Here's how the part is built. I have some questions about the finished solid (model axes, mm). A direction names the side the tool comes from. Coordinates: 2 decimals unless noted, no trailing zeros. Write each loop counter-clockwise with the first axis right and the second up, starting at its lowest first coordinate (ties: lowest second). Pieces come first, ordered by that corner, then holes. Notation, with made-up numbers: (-23, 41.5) -> (17, 41.5) arc R25 ccw to (17, 72.5) -> close; hole circle Ø2 at (6, 72). An arc over 180 degrees is marked (long way). Use a Markdown table: item, result. Add a question column.
Item 1: Imagine slicing it at C-C, the plane z = 16. Write out the boundary of the cut face in (x, y).
Item 2: Imagine slicing it at D-D, the plane z = 33.5. Write out the boundary of the cut face in (x, y), and give its area (3 significant figures).
Item 3: On a 3-axis mill with a long thin cutter (end or side, diameter ignored), from which of +Z, -Z, +X, -X, +Y, -Y can I reach the whole of each face in a straight line? I mean faces 1 (the flat face through (-45, 60, -15)), 2 (the flat face through (-6.604, 44.79, 42.767)). Say none if no direction works.
Item 4: If I drill on line 1 along Z through (x, y) = (22.5, 42.5); line 2 along X through (y, z) = (48, 29.5); line 3 along Z through (x, y) = (22, 42), over which ranges is the centre line in solid material (lowest first)? Write a range as from..to.
Item 5: Will these pins go through, and if not, where does the flat tip stop? pin 1 Ø21 at (x, z) = (-36, 9.5) entering from +Y; pin 2 Ø2 at (x, y) = (-26, 18) entering from +Z; pin 3 Ø1 at (x, y) = (1, 31.5) entering from -Z; pin 4 Ø5 at (x, y) = (-27, 41.5) entering from +Z.
Item 6: Imagine slicing it at A-A, the plane y = 54. Count the separate pieces of the cut face and the enclosed holes in it, and give its area (3 significant figures).
Item 7: Imagine slicing it at B-B, the plane y = 17.5. Write out the boundary of the cut face in (x, z), and give its area (3 significant figures).
Item 8: If we mould it in two halves opening along X, with no side actions, what happens to faces 3 (the flat face through (-33.736, 44.79, -27.102)), 4 (the flat face through (35, 60, -35)), 5 (the flat face through (-40.339, 44.79, 15.665))? For each: pulls with the +X half, pulls with the -X half, needs draft (parallel to the pull), parting line crosses it, or undercut.
```python
from build123d import *

# Parameters (mm, degrees)
BOSS_EXTRUDE1_DEPTH   = 60
BOSS_EXTRUDE1_2_DEPTH = 60
BOSS_EXTRUDE1_3_DEPTH = 60
BOSS_EXTRUDE1_4_DEPTH = 60
BOSS_EXTRUDE1_5_DEPTH = 60
BOSS_EXTRUDE1_6_DEPTH = 60
BOSS_EXTRUDE2_DEPTH   = 30


with BuildPart() as part:
    # Sketch2 → Boss-Extrude1 (new body)
    with BuildSketch(Plane(origin=(0, 0, 0), x_dir=(1, 0, 0), z_dir=(0, 1, 0))):
        with BuildLine():
            Line((18.030501156, -69.282032303), (39.961980888, -47.664077799))
            Line((39.961980888, -47.664077799), (13.634472037, -20.954741045))
            ThreePointArc((13.634472037, -20.954741045), (6.29646333, -24.194101544), (-1.689726767, -24.942831103))
            Line((-1.689726767, -24.942831103), (-11.656936488, -61.097790964))
            Line((-11.656936488, -61.097790964), (18.030501156, -69.282032303))
        make_face()
    extrude(amount=BOSS_EXTRUDE1_DEPTH)



with BuildPart() as body_2:
    # Sketch2 → Boss-Extrude1 2 (new body)
    with BuildSketch(Plane(origin=(0, 0, 0), x_dir=(1, 0, 0), z_dir=(0, 1, 0))):
        with BuildLine():
            Line((-21.297311778, -58.440129534), (-11.330102056, -22.285169674))
            ThreePointArc((-11.330102056, -22.285169674), (-17.804474894, -17.54994797), (-22.445988761, -11.008069246))
            Line((-22.445988761, -11.008069246), (-58.740707334, -20.453692353))
            Line((-58.740707334, -20.453692353), (-50.984749422, -50.255888195))
            Line((-50.984749422, -50.255888195), (-21.297311778, -58.440129534))
        make_face()
    extrude(amount=BOSS_EXTRUDE1_2_DEPTH)


with BuildPart() as body_3:
    # Sketch2 → Boss-Extrude1 3 (new body)
    with BuildSketch(Plane(origin=(0, 0, 0), x_dir=(1, 0, 0), z_dir=(0, 1, 0))):
        with BuildLine():
            ThreePointArc((-24.964574093, -1.330428629), (-24.100938224, 6.644153574), (-20.756261995, 13.934761857))
            Line((-20.756261995, 13.934761857), (-47.083770846, 40.644098611))
            Line((-47.083770846, 40.644098611), (-69.015250578, 19.026144108))
            Line((-69.015250578, 19.026144108), (-61.259292666, -10.776051735))
            Line((-61.259292666, -10.776051735), (-24.964574093, -1.330428629))
        make_face()
    extrude(amount=BOSS_EXTRUDE1_3_DEPTH)


with BuildPart() as body_4:
    # Sketch2 → Boss-Extrude1 4 (new body)
    with BuildSketch(Plane(origin=(0, 0, 0), x_dir=(1, 0, 0), z_dir=(0, 1, 0))):
        with BuildLine():
            ThreePointArc((-13.634472037, 20.954741045), (-6.29646333, 24.194101544), (1.689726767, 24.942831103))
            Line((1.689726767, 24.942831103), (11.656936488, 61.097790964))
            Line((11.656936488, 61.097790964), (-18.030501156, 69.282032303))
            Line((-18.030501156, 69.282032303), (-39.961980888, 47.664077799))
            Line((-39.961980888, 47.664077799), (-13.634472037, 20.954741045))
        make_face()
    extrude(amount=BOSS_EXTRUDE1_4_DEPTH)


with BuildPart() as body_5:
    # Sketch2 → Boss-Extrude1 5 (new body)
    with BuildSketch(Plane(origin=(0, 0, 0), x_dir=(1, 0, 0), z_dir=(0, 1, 0))):
        with BuildLine():
            Line((22.445988761, 11.008069246), (58.740707334, 20.453692353))
            Line((58.740707334, 20.453692353), (50.984749422, 50.255888195))
            Line((50.984749422, 50.255888195), (21.297311778, 58.440129534))
            Line((21.297311778, 58.440129534), (11.330102056, 22.285169674))
            ThreePointArc((11.330102056, 22.285169674), (17.804474894, 17.54994797), (22.445988761, 11.008069246))
        make_face()
    extrude(amount=BOSS_EXTRUDE1_5_DEPTH)


with BuildPart() as body_6:
    # Sketch2 → Boss-Extrude1 6 (new body)
    with BuildSketch(Plane(origin=(0, 0, 0), x_dir=(1, 0, 0), z_dir=(0, 1, 0))):
        with BuildLine():
            Line((69.015250578, -19.026144108), (61.259292666, 10.776051735))
            Line((61.259292666, 10.776051735), (24.964574093, 1.330428629))
            ThreePointArc((24.964574093, 1.330428629), (24.991141954, 0.665450098), (25, 0))
            ThreePointArc((25, 0), (23.91554463, -7.283318273), (20.756261995, -13.934761857))
            Line((20.756261995, -13.934761857), (47.083770846, -40.644098611))
            Line((47.083770846, -40.644098611), (69.015250578, -19.026144108))
        make_face()
    extrude(amount=BOSS_EXTRUDE1_6_DEPTH)


with BuildPart() as part_1:
    add(part.part)

    add(body_2.part)  # Boss-Extrude2 merges body 2

    add(body_3.part)  # Boss-Extrude2 merges body 3

    add(body_4.part)  # Boss-Extrude2 merges body 4

    add(body_5.part)  # Boss-Extrude2 merges body 5

    add(body_6.part)  # Boss-Extrude2 merges body 6
    # Sketch2_3 → Boss-Extrude2 (add)
    with BuildSketch(Plane(origin=(0, 0, 0), x_dir=(1, 0, 0), z_dir=(0, 1, 0))):
        with BuildLine():
            Line((-11.656936488, -61.097790964), (-1.689726767, -24.942831103))
            ThreePointArc((-1.689726767, -24.942831103), (-6.644153574, -24.100938224), (-11.330102056, -22.285169674))
            Line((-11.330102056, -22.285169674), (-21.297311778, -58.440129534))
            Line((-21.297311778, -58.440129534), (-11.656936488, -61.097790964))
        make_face()
        with BuildLine():
            Line((39.961980888, -47.664077799), (47.083770846, -40.644098611))
            Line((47.083770846, -40.644098611), (20.756261995, -13.934761857))
            ThreePointArc((20.756261995, -13.934761857), (17.54994797, -17.804474894), (13.634472037, -20.954741045))
            Line((13.634472037, -20.954741045), (39.961980888, -47.664077799))
        make_face()
        with BuildLine():
            Line((61.259292666, 10.776051735), (58.740707334, 20.453692353))
            Line((58.740707334, 20.453692353), (22.445988761, 11.008069246))
            ThreePointArc((22.445988761, 11.008069246), (24.194101544, 6.29646333), (24.964574093, 1.330428629))
            Line((24.964574093, 1.330428629), (61.259292666, 10.776051735))
        make_face()
        with BuildLine():
            ThreePointArc((1.689726767, 24.942831103), (6.644153574, 24.100938224), (11.330102056, 22.285169674))
            Line((11.330102056, 22.285169674), (21.297311778, 58.440129534))
            Line((21.297311778, 58.440129534), (11.656936488, 61.097790964))
            Line((11.656936488, 61.097790964), (1.689726767, 24.942831103))
        make_face()
        with BuildLine():
            ThreePointArc((-20.756261995, 13.934761857), (-17.54994797, 17.804474894), (-13.634472037, 20.954741045))
            Line((-13.634472037, 20.954741045), (-39.961980888, 47.664077799))
            Line((-39.961980888, 47.664077799), (-47.083770846, 40.644098611))
            Line((-47.083770846, 40.644098611), (-20.756261995, 13.934761857))
        make_face()
        with BuildLine():
            ThreePointArc((-22.445988761, -11.008069246), (-24.194101544, -6.29646333), (-24.964574093, -1.330428629))
            Line((-24.964574093, -1.330428629), (-61.259292666, -10.776051735))
            Line((-61.259292666, -10.776051735), (-58.740707334, -20.453692353))
            Line((-58.740707334, -20.453692353), (-22.445988761, -11.008069246))
        make_face()
    extrude(amount=BOSS_EXTRUDE2_DEPTH)


solid = part_1.part
```
Ans:
| question | item | result |
|---|---|---|
| 1 | outline | (-59.9, 0) -> (-19.21, 0) -> (-19.21, 60) -> (-41.63, 60) -> (-41.63, 30) -> (-59.9, 30) -> close; (19.21, 0) -> (68.23, 0) -> (68.23, 60) -> (22.79, 60) -> (22.79, 30) -> (19.21, 30) -> close |
| 2 | outline | (-55.35, 0) -> (54.33, 0) -> (54.33, 60) -> (40.04, 60) -> (40.04, 30) -> (26, 30) -> (26, 60) -> (-4.05, 60) -> (-4.05, 30) -> (-14.42, 30) -> (-14.42, 60) -> (-55.35, 60) -> close |
| 2 | area | 5,850 mm^2 |
| 3 | face 1 | +Z, -Z, +X, -X, +Y |
| 3 | face 2 | +Y |
| 4 | line 1 | z = -58.11..-11.02, 10.9..15.7, 29.95..64.88 |
| 4 | line 2 | x = -56.39..-13.32, -2.95..22.06, 36.1..58.39 |
| 4 | line 3 | z = -58.25..-11.87, 11.87..15.2, 29.44..65.37 |
| 5 | pin 1 | stops at y = 60 |
| 5 | pin 2 | stops at z = 57.42 |
| 5 | pin 3 | stops at z = -64.17 |
| 5 | pin 4 | stops at z = 57.56 |
| 6 | separate pieces | 6 |
| 6 | enclosed holes | 0 |
| 6 | area | 9,120 mm^2 |
| 7 | outline | (-69.02, -19.03) -> (-18.03, -69.28) -> (50.98, -50.26) -> (69.02, 19.03) -> (18.03, 69.28) -> (-50.98, 50.26) -> close; hole circle Ø50 at (0, 0) |
| 7 | area | 11,400 mm^2 |
| 8 | face 3 | undercut |
| 8 | face 4 | needs draft |
| 8 | face 5 | pulls with the -X half |
